The model under review builds one solid part; all positions refer to its coordinate system, in mm. Face numbers are marked on the shaded views. A direction names the side the tool comes from. Round coordinates to 2 decimals unless told otherwise and drop trailing zeros. Loops run counter-clockwise (first coordinate to the right, second up) from the corner with the lowest first, then second, coordinate; pieces in that order, holes last. Notation, with made-up numbers: M -11.75,-30.5 L 36.25,-30.5 A34 cw 36.25,2.5 Z; hole C 34,16.5 d5. An arc over 180 degrees is marked long. Answer as a JSON object with one key per item and string values. Group by question number.
Item 1: Consider section C-C (y = 0). Give the boundary of the cut face in (x, z).
Item 2: To check wall thickness, follow line 1 (Z direction, x = 10, y = 0); line 2 (Y direction, x = 1, z = -0.5); line 3 (Z direction, x = 7.5, y = -2). State the ranges of each line that lie inside material, in increasing order.
Item 3: Consider section B-B (x = 4.75). Give the boundary of the cut face in (y, z), and give its area (3 significant figures).
Item 4: Tool access review of the marked faces 1 and 2: name each direction out of +Z, -Z, +X, -X, +Y, -Y from which nothing blocks a thin tool from reaching the whole face with its end or side.
Item 5: Consider section D-D (x = 15.5). Give the boundary of the cut face in (y, z), and give its area (3 significant figures).
Item 6: The part is to be moulded in two halves that separate along Y. For the marked faces 3, 4 and 5, say which applies: +Y half, -Y half, draft (parallel to the pull), parting line (faces both ways), or undercut.
Item 7: Consider section A-A (z = 0.5). Give the boundary of the cut face in (x, y).
Item 8: Insertion check: P1, Ø4, axis at x = 5, z = 0, coming from the +Y side; P2, Ø2, axis at x = 4, y = -5, coming from the -Z side; P3, Ø1.8, axis at y = -1.5, z = 1, coming from the +X side. Each pin has a flat end and moves straight along its axis. Give the tip position at first contact, or say it passes through.
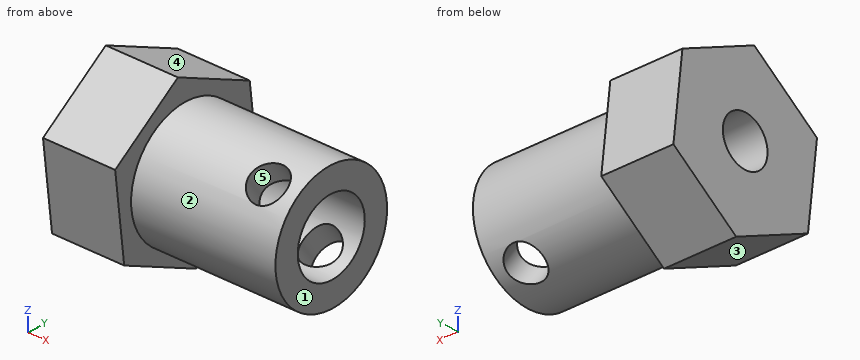
```python
from build123d import *

# Parameters (mm, degrees)
SKETCH1_R           = 5
SKETCH1_R_2         = 3
BOSS_EXTRUDE1_DEPTH = 18
BOSS_EXTRUDE2_DEPTH = 6
SKETCH3_R           = 2
CUT_EXTRUDE1_DEPTH  = 6
SKETCH4_R           = 1.5
CUT_EXTRUDE2_DEPTH  = 14


with BuildPart() as part:
    # Sketch1 → Boss-Extrude1 (new body)
    with BuildSketch(Plane(origin=(0, 0, 0), x_dir=(0, 0, -1), z_dir=(1, 0, 0))):
        Circle(SKETCH1_R)
        Circle(SKETCH1_R_2, mode=Mode.SUBTRACT)
    extrude(amount=BOSS_EXTRUDE1_DEPTH)

    # Sketch2 → Boss-Extrude2 (add)
    with BuildSketch(Plane.ZY):
        Polygon((-6.953065422, 0.809247324), (-4.177361452, -5.616907628), (2.775703971, -6.426154952), (6.953065422, -0.809247324), (4.177361452, 5.616907628), (-2.775703971, 6.426154952), align=None)
    extrude(amount=-BOSS_EXTRUDE2_DEPTH)

    # Sketch3 → Cut-Extrude1 (cut)
    with BuildSketch(Plane.ZY):
        Circle(SKETCH3_R)
    extrude(amount=-CUT_EXTRUDE1_DEPTH, mode=Mode.SUBTRACT)

    # Sketch4 → Cut-Extrude2 (cut)
    with BuildSketch(Plane(origin=(0, 3.617701138, -4.864384697), x_dir=(-1, 0, 0), z_dir=(0, 0.596765922, -0.802415375))):
        with Locations((-15.5, 0)):
            Circle(SKETCH4_R)
    extrude(amount=-CUT_EXTRUDE2_DEPTH, mode=Mode.SUBTRACT)


solid = part.part
```
Geometry results:
{
 "1": {"outline": "M 0,-6.6 L 6,-6.6 L 6,-5 L 18,-5 L 18,-3 L 6,-3 L 6,-2 L 0,-2 Z; M 0,2 L 6,2 L 6,3 L 18,3 L 18,5 L 6,5 L 6,6.6 L 0,6.6 Z"},
 "2": {"line 1": "z = -5 to -3, 3 to 5", "line 2": "y = -6.04 to -1.94, 1.94 to 6.16", "line 3": "z = -4.58 to -2.24, 2.24 to 4.58"},
 "3": {"outline": "M -6.43,2.78 L -5.62,-4.18 L 0.81,-6.95 L 6.43,-2.78 L 5.62,4.18 L -0.81,6.95 Z; hole C 0,0 d4", "area": "115 mm^2"},
 "4": {"face 1": "+Z, -Z, +X, +Y, -Y", "face 2": "+X"},
 "5": {"outline": "M -4.05,2.93 A5 ccw 1.64,-4.72 L 0.35,-2.98 A3 cw -2.75,1.19 Z; M -1.64,4.72 L -0.35,2.98 A3 cw 2.75,-1.19 L 4.05,-2.93 A5 ccw Z", "area": "37.9 mm^2"},
 "6": {"face 3": "-Y half", "face 4": "+Y half", "face 5": "undercut"},
 "7": {"outline": "M 0,-6.16 L 6,-6.16 L 6,-4.97 L 18,-4.97 L 18,-2.96 L 6,-2.96 L 6,-1.94 L 0,-1.94 Z; M 0,1.94 L 6,1.94 L 6,2.96 L 18,2.96 L 18,4.97 L 6,4.97 L 6,6.04 L 0,6.04 Z"},
 "8": {"P1": "stops at y = 6.34", "P2": "stops at z = -4.88", "P3": "stops at x = 6"}
}
